Can you work these out from the model? Positions are in its coordinate system, mm. Face numbers are marked on the shaded views. A direction names the side the tool comes from. Round coordinates to 2 decimals unless told otherwise and drop trailing zeros. Write each loop counter-clockwise with the first axis right and the second up, starting at its lowest first coordinate (ties: lowest second). Pieces come first, ordered by that corner, then holes. Notation, with made-up numbers: M 15.5,-7 L 57.5,-7 A20 cw 57.5,25 Z; hole C 25.5,-2 d8. An arc over 180 degrees is marked long. Answer in a Markdown table with one row per item. Add a question column.
(1) Suppose I cut it at C-C, the plane x = -17. Write out the boundary of the cut face in (y, z).
(2) If I drill on probe 1 along Z at (x, y) = (0, -29.5); probe 2 along Z at (x, y) = (17, 1.2); probe 3 along Y at (x, z) = (-12, 20.5), over which ranges is the centre line in solid material (lowest first)?
(3) Suppose I cut it at D-D, the plane z = 13. Write out the boundary of the cut face in (x, y).
(4) If we mould it in two halves opening along Z, with no side actions, what happens to the marked faces 4, 5 and 6? For each: released by +Z, released by -Z, zero draft, split by the parting line, or undercut.
(5) Suppose I cut it at B-B, the plane y = -1. Write out the boundary of the cut face in (x, z), then the cut area to 3 significant figures.
(6) I'm going to push flat-ended pins straight in: pin 1 (5 mm diameter, centred on x = 9.5, y = -45.5, fed in from -Z); pin 2 (2 mm diameter, centred on x = -3, z = 22, fed in from -Y); pin 3 (3.5 mm diameter, centred on x = 17, z = -0.5, fed in from -Y); pin 4 (2 mm diameter, centred on x = -17, z = -0.5, fed in from -Y). Where does each tip first touch, or does it pass through?
(7) Suppose I cut it at A-A, the plane x = 0. Write out the boundary of the cut face in (y, z), then the cut area to 3 significant figures.
(8) For the marked faces 1, 2 and 3, which set-ups out of +Z, -Z, +X, -X, +Y, -Y let a thin tool reach every point of the face, with its end or its side?
Autodesk Inventor part; units mm, degrees
ref_plane "YZ Plane" through (0, 0, 0) normal (1, 0, 0) x (0, 1, 0)
ref_plane "XZ Plane" through (0, 0, 0) normal (0, 1, 0) x (-1, 0, 0)
ref_plane "XY Plane" through (0, 0, 0) normal (0, 0, 1) x (1, 0, 0)
sketch "Esboço1" plane through (0, 0, 0) normal (0, 1, 0) x (-1, 0, 0)
  line L0 (24, 28) -> (-24, 28)
  line L1 (-24, 28) -> (-24, -28)
  line L2 (-24, -28) -> (24, -28)
  line L3 (24, -28) -> (24, 28)
  line L4 (24, 28) -> (-24, -28) construction
  line L5 (-24, 28) -> (24, -28) construction
  point P0 (0, 0)
  dimension "d0" = 48
  dimension "d1" = 56
extrude "Base" add sketch "Esboço1" along normal blind 3
sketch "Esboço2" plane through (0, 3, 0) normal (0, 1, 0) x (1, 0, 0)
  line L0 (-20.5, -25) -> (20.5, -25)
  line L1 (20.5, -25) -> (20.5, 25)
  line L2 (20.5, 25) -> (-20.5, 25)
  line L3 (-20.5, 25) -> (-20.5, -25)
  line L4 (-20.5, -25) -> (20.5, 25) construction
  line L5 (20.5, -25) -> (-20.5, 25) construction
  line L6 (-24, 28) -> (-24, -28)
  point P0 (0, 0)
  dimension "d4" = 41
  dimension "d5" = 50
extrude "Encaixe" add sketch "Esboço2" along normal blind 2
ref_plane "Plano de trabalho2" through (0, 0, -28) normal (-1, 0, 0) x (0, 0, 1)
sketch "Esboço9" plane through (0, 0, 0) normal (0, -1, 0) x (1, 0, 0)
  line L0 (9.8995, 0) -> (0, -9.8995)
  line L1 (0, -9.8995) -> (-9.8995, 0)
  line L2 (-9.8995, 0) -> (0, 9.8995)
  line L3 (0, 9.8995) -> (9.8995, 0)
  point P0 (0, 0)
  point P1 (0, 0)
  dimension "d33" = 14
extrude "Extrusão7" add sketch "Esboço9" along normal blind 80
sketch "Esboço10" plane through (0, -80, 0) normal (0, -1, 0) x (1, 0, 0)
  circle A0 centre (0, 0) radius 3.5
  dimension "d36" = 7
extrude "Extrusão8" cut sketch "Esboço10" against normal up to surface (85 mm away)
fillet "Arredondamento1" radius 2 4 edges at (-9.8995, -40, 0) (0, -40, -9.8995) (9.8995, -40, 0) (0, -40, 9.8995)
sketch "Esboço11" plane through (0, 0, 0) normal (0, -1, 0) x (1, 0, 0)
  circle A0 centre (-17, -0.5) radius 1.1
  circle A1 centre (17, -0.5) radius 1.1
  line L0 (-24, -28) -> (-24, 28)
  line L1 (24, 28) -> (24, -28)
  line L2 (24, -28) -> (-24, -28)
  point P0 (0, 0)
  dimension "d40" = 2.2
  dimension "d41" = 2.2
  dimension "d42" = 7
  dimension "d43" = 7
  dimension "d44" = 27.5
  dimension "d45" = 27.5
extrude "Extrusão9" cut sketch "Esboço11" against normal up to next
sketch "Esboço12" plane through (0, 0, 0) normal (0, -1, 0) x (1, 0, 0)
  circle A0 centre (-17, -0.5) radius 1.1
  circle A1 centre (-17, -0.5) radius 2.6
  circle A2 centre (17, -0.5) radius 1.1
  circle A3 centre (17, -0.5) radius 2.6
  point P0 (0, 0)
  dimension "d48" = 5.2
  dimension "d49" = 5.2
extrude "Extrusão10" cut sketch "Esboço12" against normal blind 3
properties part number "Tampa Eletroimã_3DPrint"
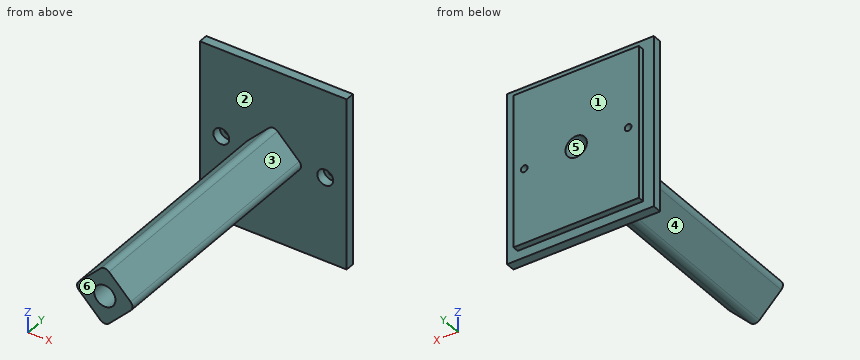
Calculated:
| question | item | result |
|---|---|---|
| 1 | outline | M 0,-28 L 3,-28 L 3,-25 L 5,-25 L 5,-1.6 L 3,-1.6 L 3,-3.1 L 0,-3.1 Z; M 0,2.1 L 3,2.1 L 3,0.6 L 5,0.6 L 5,25 L 3,25 L 3,28 L 0,28 Z |
| 2 | probe 1 | -9.07 to -3.5, 3.5 to 9.07 |
| 2 | probe 2 | -28 to -3.1, 2.1 to 28 |
| 2 | probe 3 | 0 to 5 |
| 3 | outline | M -24,0 L 24,0 L 24,3 L 20.5,3 L 20.5,5 L -20.5,5 L -20.5,3 L -24,3 Z |
| 4 | face 4 | released by -Z |
| 4 | face 5 | undercut |
| 4 | face 6 | zero draft |
| 5 | outline | M -8.49,-1.41 L -1.41,-8.49 A2 ccw 1.41,-8.49 L 8.49,-1.41 A2 ccw 8.49,1.41 L 1.41,8.49 A2 ccw -1.41,8.49 L -8.49,1.41 A2 ccw Z; hole C 0,0 d7 |
| 5 | area | 154 mm² |
| 6 | pin 1 | z = -2.9 |
| 6 | pin 2 | y = 0 |
| 6 | pin 3 | y = 3 |
| 6 | pin 4 | through |
| 7 | outline | M -80,-9.07 L 0,-9.07 L 0,-28 L 3,-28 L 3,-25 L 5,-25 L 5,-3.5 L -80,-3.5 Z; M -80,3.5 L 5,3.5 L 5,25 L 3,25 L 3,28 L 0,28 L 0,9.07 L -80,9.07 Z |
| 7 | area | 1,120 mm² |
| 8 | face 1 | +Z, -Z, +X, -X, +Y |
| 8 | face 2 | -Y |
| 8 | face 3 | +Z, +X, -Y |
